from build123d import *

# Parameters (mm, degrees)
SKETCH1_W           = 91.44
SKETCH1_H           = 91.44
BOSS_EXTRUDE1_DEPTH = 3.175
SKETCH2_R           = 38.1
BOSS_EXTRUDE2_DEPTH = 2.54
SKETCH4_R           = 1.143
BOSS_EXTRUDE4_DEPTH = 5.08
SKETCH5_R           = 1.143
BOSS_EXTRUDE5_DEPTH = 5.08


with BuildPart() as part:
    # Sketch1 → Boss-Extrude1 (new body)
    with BuildSketch(Plane(origin=(0, 0, 0), x_dir=(1, 0, 0), z_dir=(0, 1, 0))):
        with Locations((32.163488372, -2.791046512)):
            Rectangle(SKETCH1_W, SKETCH1_H)
    extrude(amount=BOSS_EXTRUDE1_DEPTH)

    # Sketch2 → Boss-Extrude2 (add)
    with BuildSketch(Plane(origin=(0, 3.175, 0), x_dir=(1, 0, 0), z_dir=(0, 1, 0))):
        with Locations(Location((32.163488372, -2.791046512, 0), (0, 0, 270))):
            Circle(SKETCH2_R)
    extrude(amount=BOSS_EXTRUDE2_DEPTH)

    # Sketch4 → Boss-Extrude4 (add)
    with BuildSketch(Plane(origin=(0, 3.175, 0), x_dir=(1, 0, 0), z_dir=(0, 1, 0))):
        with Locations(Location((9.303488372, -43.431046512, 0), (0, 0, 270))):
            Circle(SKETCH4_R)
        with Locations(Location((57.563488372, -43.431046512, 0), (0, 0, 270))):
            Circle(SKETCH4_R)
    extrude(amount=BOSS_EXTRUDE4_DEPTH)

    # Sketch5 → Boss-Extrude5 (add)
    with BuildSketch(Plane(origin=(0, 3.175, 0), x_dir=(1, 0, 0), z_dir=(0, 1, 0))):
        with Locations(Location((-8.476511628, 37.848953488, 0), (0, 0, 270))):
            Circle(SKETCH5_R)
        with Locations(Location((72.803488372, 37.848953488, 0), (0, 0, 270))):
            Circle(SKETCH5_R)
    extrude(amount=BOSS_EXTRUDE5_DEPTH)


solid = part.part
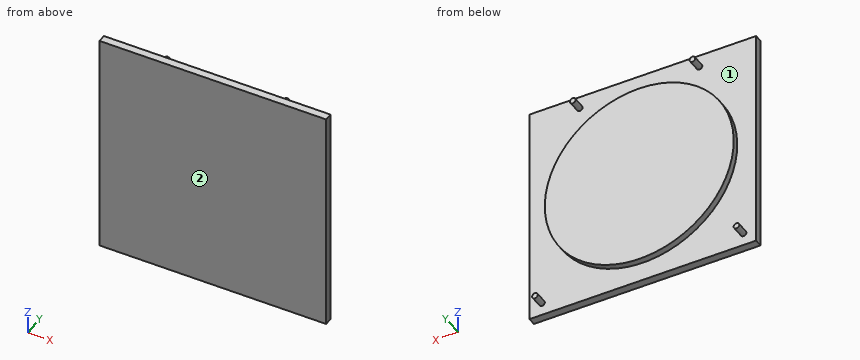
Could you check a few things on this model? Use its own coordinates, in mm. Face numbers are marked on the shaded views. A direction names the side the tool comes from. Coordinates: 2 decimals unless noted, no trailing zeros. Order: outer loops, then holes, each group sorted by start corner. A loop starts at its lowest first (then second) coordinate and runs counter-clockwise, first axis right, second up. Notation, with made-up numbers: (57.5, -21.5) -> (95.5, -21.5) arc R37 cw to (95.5, 14.5) -> close; hole circle Ø11 at (85, 48). An arc over 180 degrees is marked (long way). One line per question, with ' | ' between items.
Q1. I'm going to push a flat-ended pin straight in: P1, Ø2, axis at x = 50, z = 17, coming from the +Y side (3 decimals). Where does the tip first touch, or does it pass through?
Return value:
P1: y = 5.715
Q2. Imagine slicing it at A-A on x = 47. Please give me the cut outline in (y, z) (3 decimals).
Return value:
outline: (0, -42.929) -> (3.175, -42.929) -> (3.175, -32.302) -> (5.715, -32.302) -> (5.715, 37.884) -> (3.175, 37.884) -> (3.175, 48.511) -> (0, 48.511) -> close
Q3. Imagine slicing it at B-B on z = -20. Please give me the cut outline in (x, y) (3 decimals).
Return value:
outline: (-13.557, 0) -> (77.883, 0) -> (77.883, 3.175) -> (62.695, 3.175) -> (62.695, 5.715) -> (1.632, 5.715) -> (1.632, 3.175) -> (-13.557, 3.175) -> close
Q4. If I drill on L1, parallel to Y at x = 12.5, z = -5.5 (3 decimals); L2, parallel to Y at x = 17.5, z = -38.5 (3 decimals); L3, parallel to X at y = 4.75, z = 43, over which ranges is the centre line in solid material (lowest first)?
Return value:
L1: 0 to 5.715 | L2: 0 to 3.175 | L3: 8.24 to 10.36, 56.5 to 58.62
Q5. On a 3-axis mill with a long thin cutter (end or side, diameter ignored), from which of +Z, -Z, +X, -X, +Y, -Y can I reach the whole of each face in a straight line? I mean the marked faces 1 and 2. Say none if no direction works.
Return value:
face 1: +Y | face 2: +Z, -Z, +X, -X, -Y
